```python
from build123d import *

# Parameters (mm, degrees)
F0_W      = 151.3425782323
F0_H      = 172.1224486828
F1_DEPTH  = 127
F3_W      = 34.7741246223
F3_H      = 30.3159058094
F4_DEPTH  = 50.8
F5_W      = 14.7121287882
F5_H      = 17.3870623112
F6_DEPTH  = 25.4
F7_R      = 34.2587493425
F8_DEPTH  = 76.2
F10_DEPTH = 177.8
F13_DEPTH = 49.276
F14_W     = 71.1912401021
F14_H     = 73.1580201536
F15_DEPTH = 189.385448
F16_W     = 95.4910255969
F16_H     = 96.0185993463
F17_DEPTH = 508
F18_R     = 22.6550220724
F19_DEPTH = 25.4
F20_R     = 12.5097530491
F21_DEPTH = 25.4
F22_R     = 13.338874827
F23_DEPTH = 25.4
F24_R     = 6.9241134555
F25_DEPTH = 25.4


with BuildPart() as f1:
    # F0 (on Top) → F1 (new body)
    with BuildSketch(Plane.XY):
        with Locations((3.3693946898, -86.0612243414)):
            Rectangle(F0_W, F0_H)
    extrude(amount=F1_DEPTH)

    # F3 (on face) → F4 (cut)
    with BuildSketch(Plane.YZ.offset(79.0406838059)):
        with Locations((-144.2410051823, 98.4970331192)):
            Rectangle(F3_W, F3_H)
    extrude(amount=-F4_DEPTH, mode=Mode.SUBTRACT)

    # F5 (on face) → F6 (cut)
    with BuildSketch(Plane.XY.offset(127)):
        with Locations((27.4437833577, -151.5970826149)):
            Rectangle(F5_W, F5_H)
    extrude(amount=-F6_DEPTH, mode=Mode.SUBTRACT)

    # F7 (on face) → F8 (cut)
    with BuildSketch(Plane(origin=(0, 0, 0), x_dir=(-1, 0, 0), z_dir=(0, 1, 0))):
        with Locations((-6.7130560055, 86.9056582451)):
            Circle(F7_R)
    extrude(amount=-F8_DEPTH, mode=Mode.SUBTRACT)

    # F9 (on face) → F10 (join)
    with BuildSketch(Plane(origin=(-72.3018944263, 0, 0), x_dir=(0, -1, 0), z_dir=(-1, 0, 0))):
        Polygon((68.4512555599, 76.6869447389), (68.4512555599, 90.8828713736), (60.1070992414, 102.3676172721), (46.6059707105, 106.7543998531), (33.1048421797, 102.3676172721), (24.7606858611, 90.8828713736), (24.7606858611, 76.6869447389), (33.1048421797, 65.2021988404), (46.6059707105, 60.8154162594), (60.1070992414, 65.2021988404), align=None)
    extrude(amount=F10_DEPTH)

    # F12 (on face) → F13 (join)
    with BuildSketch(Plane(origin=(0, -76.2, 0), x_dir=(-1, 0, 0), z_dir=(0, 1, 0))):
        Polygon((4.7714961833, 79.0930910356), (10.800817036, 87.215729212), (10.9042731407, 97.3310274144), (5.0423477816, 105.5752855359), (-4.5459027936, 108.7994771861), (-14.1980927578, 105.7720707409), (-20.2274136105, 97.6494325645), (-20.3308697152, 87.5341343621), (-14.4689443561, 79.2898762406), (-4.8806937809, 76.0656845904), align=None)
    extrude(amount=F13_DEPTH)

    # F14 (on face) → F15 (cut)
    with BuildSketch(Plane.YZ.offset(79.0406838059)):
        with Locations((-47.7073919028, 55.1417870447)):
            Rectangle(F14_W, F14_H)
    extrude(amount=-F15_DEPTH, mode=Mode.SUBTRACT)

    # F16 (on face) → F17 (join)
    with BuildSketch(Plane.XY.offset(127)):
        with Locations((5.4796915501, -69.1788261756)):
            Rectangle(F16_W, F16_H)
    extrude(amount=F17_DEPTH)

    # F18 (on face) → F19 (cut)
    with BuildSketch(Plane(origin=(0, -21.1695265025, 0), x_dir=(-1, 0, 0), z_dir=(0, 1, 0))):
        with Locations((-23.0861343443, 237.3967021704)):
            Circle(F18_R)
    extrude(amount=-F19_DEPTH, mode=Mode.SUBTRACT)

    # F20 (on face) → F21 (join)
    with BuildSketch(Plane(origin=(0, -46.5695265025, 0), x_dir=(-1, 0, 0), z_dir=(0, 1, 0))):
        with Locations((-23.0861343443, 237.3967021704)):
            Circle(F20_R)
    extrude(amount=-F21_DEPTH)

    # F22 (on face) → F23 (join)
    with BuildSketch(Plane(origin=(0, -46.5695265025, 0), x_dir=(-1, 0, 0), z_dir=(0, 1, 0))):
        with Locations((-23.0861343443, 237.3967021704)):
            Circle(F22_R)
    extrude(amount=F23_DEPTH)

    # F24 (on face) → F25 (join)
    with BuildSketch(Plane(origin=(0, -21.1695265025, 0), x_dir=(-1, 0, 0), z_dir=(0, 1, 0))):
        with Locations((-23.0861343443, 237.3967021704)):
            Circle(F24_R)
    extrude(amount=F25_DEPTH)


solid = f1.part
```
Source: CAD feature listing. Evaluate the final solid. Frame: model axes, mm. A direction names the side the tool comes from. Give positions to 0.01 mm unless a question says otherwise; leave off trailing zeros. Write each loop counter-clockwise with the first axis right and the second up, starting at its lowest first coordinate (ties: lowest second). Pieces come first, ordered by that corner, then holes. Notation, with made-up numbers: (-25, -25) - (-17, -25) arc R32 ccw to (-17, 1) - close; hole circle Ø11 at (88, -36). An arc over 180 degrees is marked (long way). One line per item, written item: value. Start each with the question number.
Q1. Section query B-B, the plane x = -191. Return the cut outline in (y, z).
Q2. Section query C-C, the plane z = 326.5. Return the cut outline in (x, y), then the cut area to 3 significant figures.
Q3. Set-up query: faces 5 (the face through (-159.96, -53.45, 104.53)), 6 (the face through (54, -161.628, 98)), 7 (the face through (4, -83.303, 55)), 8 (the face through (-110.345, -47, 80)), 9 (the face through (17, -21.17, 232)). Return all of +Z, -Z, +X, -X, +Y, -Y with unobstructed straight access to the full face (end or side cutting, diameter ignored); none if empty.
Q4. Section query A-A, the plane y = -110. Return the cut outline in (x, z).
Q5. Material intervals for probe 1 along X at (y, z) = (-43.5, 85); probe 2 along X at (y, z) = (-54.5, 249); probe 3 along Z at (x, y) = (8, -31), sorted ascending. Write a range as from..to.
Q6. First-contact query: pin 1 Ø4 at (y, z) = (-152, 120) entering from -X; pin 2 Ø13.5 at (x, z) = (-2.5, 101.5) entering from +Y; pin 3 Ø15.5 at (y, z) = (-54.5, 81) entering from +X. Flat tips, straight axial feed; report the tip coordinate or a pass-through.
Q7. Draft query along X for faces 1 (the face through (5, -117.188, 377)), 2 (the face through (20.088, -152, 114)), 3 (the face through (-11.704, -37.567, 115.793)), 4 (the face through (28.58, -8.65, 233.18)). Return one class per face: +X half, -X half, draft (parallel to the pull), parting line (faces both ways), or undercut.
Q8. Section query D-D, the plane x = -78.5. Return the cut outline in (y, z), then the cut area to 3 significant figures.
Answer:
1. outline: (-68.45, 76.69) - (-60.11, 65.2) - (-46.61, 60.82) - (-33.1, 65.2) - (-24.76, 76.69) - (-24.76, 90.88) - (-33.1, 102.37) - (-46.61, 106.75) - (-60.11, 102.37) - (-68.45, 90.88) - close
2. outline: (-42.27, -117.19) - (53.23, -117.19) - (53.23, -21.17) - (-42.27, -21.17) - close
2. area: 9,170 mm2
3. face 5: +Z, -X, -Y
3. face 6: +X
3. face 7: +X, -X
3. face 8: -Z, +X, +Y, -Y
3. face 9: +Y
4. outline: (-72.3, 0) - (79.04, 0) - (79.04, 127) - (53.23, 127) - (53.23, 635) - (-42.27, 635) - (-42.27, 127) - (-72.3, 127) - close
5. probe 1: x = -250.1..-110.34
5. probe 2: x = -42.27..53.23
5. probe 3: z = 0..18.56, 91.72..107.72, 121.14..220.5, 254.3..635
6. pin 1: stops at x = -72.3
6. pin 2: stops at y = -26.92
6. pin 3: stops at x = -110.34
7. face 1: draft
7. face 2: undercut
7. face 3: undercut
7. face 4: parting line
8. outline: (-67.84, 91.72) - (-25.37, 91.72) - (-33.1, 102.37) - (-46.61, 106.75) - (-60.11, 102.37) - close
8. area: 429 mm2
